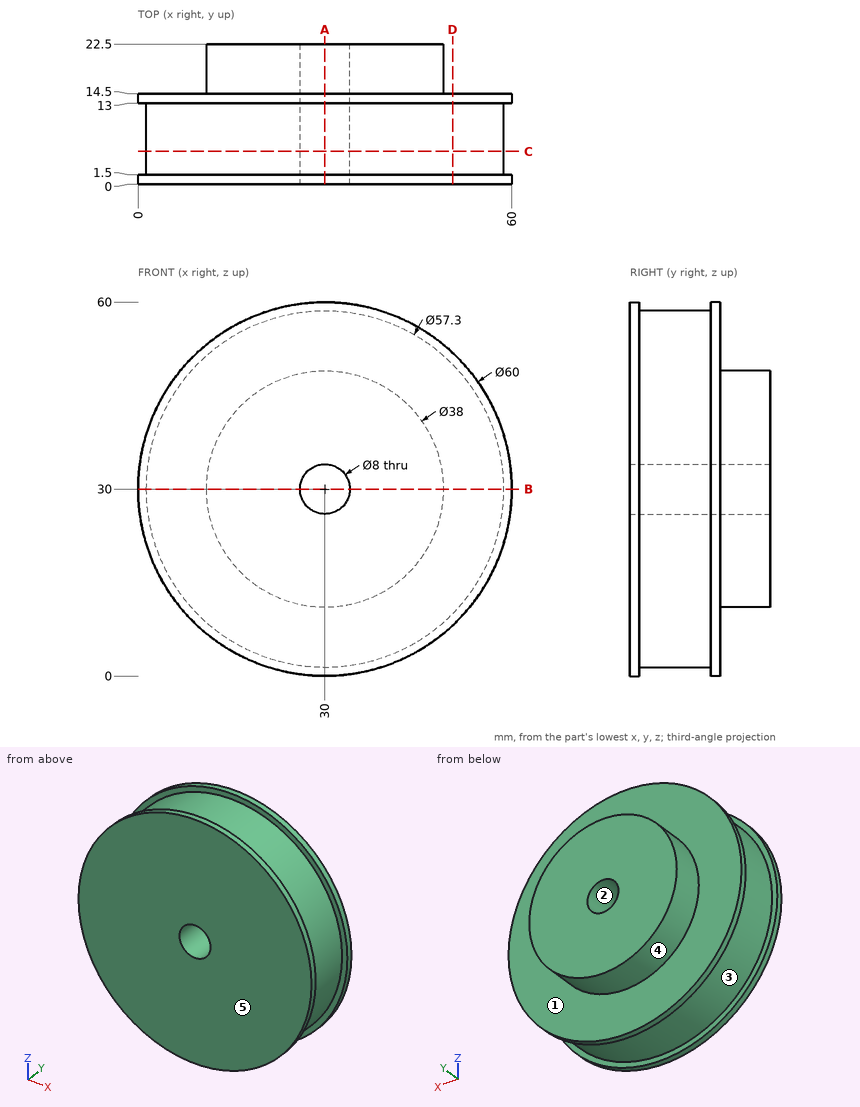
Source: three-view drawing plus pictorial views. Frame: mm from the lowest corner of the part. A direction names the side the tool comes from. Give positions to 0.01 mm unless a question says otherwise; leave off trailing zeros. Order: outer loops, then holes, each group sorted by start corner. A loop starts at its lowest first (then second) coordinate and runs counter-clockwise, first axis right, second up.
1. Section B-B on z = 30. Return the cut outline in (x, y), and give its area (3 significant figures).
Derived:
outline: (0, 0) - (26, 0) - (26, 22.5) - (11, 22.5) - (11, 14.5) - (0, 14.5) - (0, 13) - (1.35, 13) - (1.35, 1.5) - (0, 1.5) - close; (34, 0) - (60, 0) - (60, 1.5) - (58.65, 1.5) - (58.65, 13) - (60, 13) - (60, 14.5) - (49, 14.5) - (49, 22.5) - (34, 22.5) - close
area: 963 mm2
2. Material intervals for L1, parallel to Z at x = 30, y = 17.25; L2, parallel to Y at x = 53, z = 13; L3, parallel to Z at x = 30, y = 5, sorted ascending.
Derived:
L1: z = 11 to 26, 34 to 49
L2: y = 0 to 14.5
L3: z = 1.35 to 26, 34 to 58.65
3. Reachability of the marked faces 4 and 5 from +Z, -Z, +X, -X, +Y, -Y: full face, straight path, thin tool, end or side. Return the list, or none.
Derived:
face 4: +Y
face 5: +Z, -Z, +X, -X, -Y
4. Pin query (flat end, axial travel): pin 1 (5 mm diameter, centred on y = 20, z = 14, fed in from -X); pin 2 (1.5 mm diameter, centred on x = 50, y = 19.5, fed in from -Z); pin 3 (6 mm diameter, centred on x = 41.5, y = 16.5, fed in from +Z); pin 4 (5 mm diameter, centred on x = 41.5, y = 11, fed in from -Z). Return the tip coordinate at first contact, or that it passes through.
Derived:
pin 1: stops at x = 16.63
pin 2: passes through
pin 3: stops at z = 58.53
pin 4: stops at z = 1.72
5. Mould query, pull axis X, two halves, no side actions, for the marked faces 1, 2 and 3. Classes: released by +X, released by -X, zero draft, split by the parting line, or undercut.
Derived:
face 1: zero draft
face 2: undercut
face 3: split by the parting line
6. Section D-D on x = 50.5. Return the cut outline in (y, z).
Derived:
outline: (0, 8.1) - (1.5, 8.1) - (1.5, 9.99) - (13, 9.99) - (13, 8.1) - (14.5, 8.1) - (14.5, 51.9) - (13, 51.9) - (13, 50.01) - (1.5, 50.01) - (1.5, 51.9) - (0, 51.9) - close
7. Section A-A on x = 30. Return the cut outline in (y, z).
Derived:
outline: (0, 0) - (1.5, 0) - (1.5, 1.35) - (13, 1.35) - (13, 0) - (14.5, 0) - (14.5, 11) - (22.5, 11) - (22.5, 26) - (0, 26) - close; (0, 34) - (22.5, 34) - (22.5, 49) - (14.5, 49) - (14.5, 60) - (13, 60) - (13, 58.65) - (1.5, 58.65) - (1.5, 60) - (0, 60) - close
8. Section C-C on y = 5.25. Return the cut outline in (x, z).
Derived:
outline: circle Ø57.3 at (30, 30); hole circle Ø8 at (30, 30)
